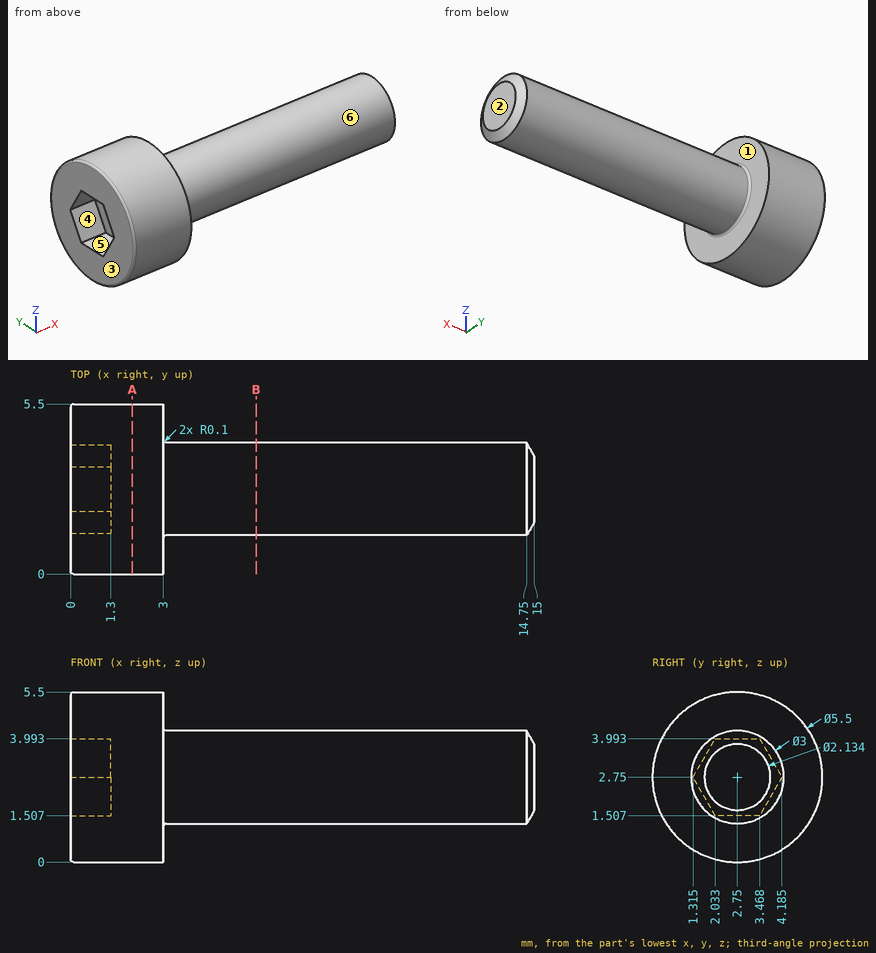
Drawing for the job (mm, zero at the part's lowest x, y, z). A direction names the side the tool comes from. Round coordinates to 2 decimals unless told otherwise and drop trailing zeros. Write each loop counter-clockwise with the first axis right and the second up, starting at its lowest first coordinate (ties: lowest second). Pieces come first, ordered by that corner, then holes. Notation, with made-up numbers: (-20.5, 39.25) - (21.5, 39.25) arc R11 ccw to (21.5, 59.25) - close; hole circle Ø11 at (25.25, 64). An arc over 180 degrees is marked (long way). Use CSV: the item, a comma, the result in double quotes.
(1) 3-axis set-ups, long thin cutter, end or side, ignore diameter. For the marked faces 1 and 2: which of +Z, -Z, +X, -X, +Y, -Y reach the whole face in a straight line?
Response:
face 1,"+X"
face 2,"+Z, -Z, +X, +Y, -Y"
(2) Band-saw the part on A-A (x = 2). Write the cut outline in (y, z).
Response:
outline,"circle Ø5.5 at (2.75, 2.75)"
(3) Mould opens along Y. For the marked faces 3, 4, 5 and 6 say: pulls with the +Y half, pulls with the -Y half, needs draft (parallel to the pull), parting line crosses it, or undercut.
Response:
face 3,"needs draft"
face 4,"undercut"
face 5,"undercut"
face 6,"parting line crosses it"
(4) Pin check, flat tips, straight feed: P1, Ø1, axis at y = 1.5, z = 1, coming from the -X side; P2, Ø1.2, axis at y = 2.5, z = 3, coming from the -X side; P3, Ø1, axis at x = 4, y = 4.5, coming from the -Z side; P4, Ø3, axis at x = 6.5, y = 1, coming from the +Z side. Stop position of each tip, or through.
Response:
P1,"x = 0"
P2,"x = 1.3"
P3,"z = 1.92"
P4,"z = 4.23"
(5) Wall check: line 1 (X direction, y = 0.8, z = 3.15); line 2 (Y direction, x = 9.5, z = 2.8). Give the ranges that are in metal, low to high.
Response:
line 1,"0 to 3"
line 2,"1.25 to 4.25"
(6) Band-saw the part on B-B (x = 6). Write the cut outline in (y, z).
Response:
outline,"circle Ø3 at (2.75, 2.75)"
